from build123d import *

# Parameters (mm, degrees)
SKETCH1_W            = 275
SKETCH1_H            = 33
BOSS_EXTRUDE1_DEPTH  = 12
CUT_EXTRUDE1_REACH   = 141.005
SKETCH2_R            = 11
SKETCH2_R_2          = 2.5
BOSS_EXTRUDE2_DEPTH  = 12
CUT_EXTRUDE2_REACH   = 250.863
SKETCH4_R            = 2.5
CUT_EXTRUDE3_REACH   = 278.522
SKETCH5_W            = 14
SKETCH5_H            = 6
FILLET1_R            = 2
FILLET1_OF_MIRROR2_R = 2
CHAMFER1_SIZE        = 10
CUT_EXTRUDE4_REACH   = 278.522
SKETCH6_W            = 12
SKETCH6_H            = 30
CHAMFER2_SIZE        = 10


with BuildPart() as part:
    # Sketch1 → Boss-Extrude1 (new body)
    with BuildSketch(Plane.XY):
        Rectangle(SKETCH1_W, SKETCH1_H)
    extrude(amount=BOSS_EXTRUDE1_DEPTH)

    # Sketch2 → Cut-Extrude1 (cut, up to next)
    with BuildSketch(Plane.XY.offset(12), mode=Mode.PRIVATE) as cut_extrude1_sk1:
        with Locations((0, 1)):
            Circle(SKETCH2_R)
    cut_extrude1_tool1 = extrude(cut_extrude1_sk1.sketch, amount=-CUT_EXTRUDE1_REACH, mode=Mode.PRIVATE) & part.part
    # Sketch2 → Cut-Extrude1 (cut, up to next)
    with BuildSketch(Plane.XY.offset(12), mode=Mode.PRIVATE) as cut_extrude1_sk2:
        with Locations((-16.5, 1)):
            Circle(SKETCH2_R_2)
    cut_extrude1_tool2 = extrude(cut_extrude1_sk2.sketch, amount=-CUT_EXTRUDE1_REACH, mode=Mode.PRIVATE) & part.part
    # Sketch2 → Cut-Extrude1 (cut, up to next)
    with BuildSketch(Plane.XY.offset(12), mode=Mode.PRIVATE) as cut_extrude1_sk3:
        with Locations((16.5, 1)):
            Circle(SKETCH2_R_2)
    cut_extrude1_tool3 = extrude(cut_extrude1_sk3.sketch, amount=-CUT_EXTRUDE1_REACH, mode=Mode.PRIVATE) & part.part
    add(cut_extrude1_tool1.solids().sort_by_distance((0, 1, 12))[0], mode=Mode.SUBTRACT)
    add(cut_extrude1_tool2.solids().sort_by_distance((-16.5, 1, 12))[0], mode=Mode.SUBTRACT)
    add(cut_extrude1_tool3.solids().sort_by_distance((16.5, 1, 12))[0], mode=Mode.SUBTRACT)

    # Sketch3 → Boss-Extrude2 (add)
    with BuildSketch(Plane.XY.offset(12)):
        Polygon((-210, 16.5), (210, 16.5), (210, 179.5), (183, 179.5), (183, 46.5), (-183, 46.5), (-183, 179.5), (-210, 179.5), align=None)
    extrude(amount=-BOSS_EXTRUDE2_DEPTH)

    # Sketch4 → Cut-Extrude2 (cut, up to next)
    with BuildSketch(Plane(origin=(0, 46.5, 0), x_dir=(1, 0, 0), z_dir=(0, 1, 0)), mode=Mode.PRIVATE) as cut_extrude2_sk1:
        with Locations(Location((-144, -6, 0), (0, 0, 270))):
            Circle(SKETCH4_R)
    cut_extrude2_tool1 = extrude(cut_extrude2_sk1.sketch, amount=-CUT_EXTRUDE2_REACH, mode=Mode.PRIVATE) & part.part
    # Sketch4 → Cut-Extrude2 (cut, up to next)
    with BuildSketch(Plane(origin=(0, 46.5, 0), x_dir=(1, 0, 0), z_dir=(0, 1, 0)), mode=Mode.PRIVATE) as cut_extrude2_sk2:
        with Locations(Location((-176, -6, 0), (0, 0, 270))):
            Circle(SKETCH4_R)
    cut_extrude2_tool2 = extrude(cut_extrude2_sk2.sketch, amount=-CUT_EXTRUDE2_REACH, mode=Mode.PRIVATE) & part.part
    cut_extrude2_1 = cut_extrude2_tool1.solids().sort_by_distance((-144, 46.5, 6))[0]
    add(cut_extrude2_1, mode=Mode.SUBTRACT)
    cut_extrude2_2 = cut_extrude2_tool2.solids().sort_by_distance((-176, 46.5, 6))[0]
    add(cut_extrude2_2, mode=Mode.SUBTRACT)
    cut_extrude2 = cut_extrude2_1 + cut_extrude2_2  # Cut-Extrude2 as one shape, for the pattern or mirror that repeats it

    # Mirror1: Cut-Extrude2 across plane
    add(cut_extrude2.mirror(Plane(origin=(0, 0, 0), x_dir=(0, 0, 1), z_dir=(1, 0, 0))), mode=Mode.SUBTRACT)

    # Sketch5 → Cut-Extrude3 (cut, up to next)
    with BuildSketch(Plane.XY.offset(12), mode=Mode.PRIVATE) as cut_extrude3_sk1:
        with Locations((-176, 43.5)):
            Rectangle(SKETCH5_W, SKETCH5_H)
    cut_extrude3_tool1 = extrude(cut_extrude3_sk1.sketch, amount=-CUT_EXTRUDE3_REACH, mode=Mode.PRIVATE) & part.part
    # Sketch5 → Cut-Extrude3 (cut, up to next)
    with BuildSketch(Plane.XY.offset(12), mode=Mode.PRIVATE) as cut_extrude3_sk2:
        with Locations((-144, 43.5)):
            Rectangle(SKETCH5_W, SKETCH5_H)
    cut_extrude3_tool2 = extrude(cut_extrude3_sk2.sketch, amount=-CUT_EXTRUDE3_REACH, mode=Mode.PRIVATE) & part.part
    cut_extrude3_1 = cut_extrude3_tool1.solids().sort_by_distance((-176, 43.5, 12))[0]
    add(cut_extrude3_1, mode=Mode.SUBTRACT)
    cut_extrude3_2 = cut_extrude3_tool2.solids().sort_by_distance((-144, 43.5, 12))[0]
    add(cut_extrude3_2, mode=Mode.SUBTRACT)
    cut_extrude3 = cut_extrude3_1 + cut_extrude3_2  # Cut-Extrude3 as one shape, for the pattern or mirror that repeats it

    # Fillet1
    fillet1_edges = [part.edges().sort_by_distance(p)[0] for p in [
        (-169, 40.5, 6),
        (-183, 40.5, 6),
        (-137, 40.5, 6),
        (-151, 40.5, 6),
    ]]
    fillet(fillet1_edges, radius=FILLET1_R)

    # Mirror2: Cut-Extrude3 across plane
    add(cut_extrude3.mirror(Plane(origin=(0, 0, 0), x_dir=(0, 0, 1), z_dir=(1, 0, 0))), mode=Mode.SUBTRACT)

    # Fillet1 of Mirror2
    fillet1_of_mirror2_edges = [part.edges().sort_by_distance(p)[0] for p in [
        (169, 40.5, 6),
        (183, 40.5, 6),
        (137, 40.5, 6),
        (151, 40.5, 6),
    ]]
    fillet(fillet1_of_mirror2_edges, radius=FILLET1_OF_MIRROR2_R)

    # Chamfer1
    chamfer1_edges = [part.edges().sort_by_distance(p)[0] for p in [
        (210, 16.5, 6),
        (-210, 16.5, 6),
    ]]
    chamfer(chamfer1_edges, length=CHAMFER1_SIZE)

    # Sketch6 → Cut-Extrude4 (cut, up to next)
    with BuildSketch(Plane.XY.offset(12), mode=Mode.PRIVATE) as cut_extrude4_sk1:
        with Locations((-194, 164.5)):
            Rectangle(SKETCH6_W, SKETCH6_H)
    cut_extrude4_tool1 = extrude(cut_extrude4_sk1.sketch, amount=-CUT_EXTRUDE4_REACH, mode=Mode.PRIVATE) & part.part
    cut_extrude4 = cut_extrude4_tool1.solids().sort_by_distance((-194, 164.5, 12))[0]
    add(cut_extrude4, mode=Mode.SUBTRACT)

    # Mirror3: Cut-Extrude4 across plane
    add(cut_extrude4.mirror(Plane(origin=(0, 0, 0), x_dir=(0, 0, 1), z_dir=(1, 0, 0))), mode=Mode.SUBTRACT)

    # Chamfer2
    chamfer2_edges = [part.edges().sort_by_distance(p)[0] for p in [
        (210, 179.5, 6),
        (-210, 179.5, 6),
    ]]
    chamfer(chamfer2_edges, length=CHAMFER2_SIZE - 0.0001)  # a hair under: the kernel refuses the full size


solid = part.part
Build history of the part. All positions in model axes, mm. A direction names the side the tool comes from. Round coordinates to 2 decimals unless told otherwise and drop trailing zeros. Write each loop counter-clockwise with the first axis right and the second up, starting at its lowest first coordinate (ties: lowest second). Pieces come first, ordered by that corner, then holes. Notation, with made-up numbers: (36.5, 24) -> (54.5, 24) arc R32 cw to (54.5, 55) -> close; hole circle Ø5 at (51, 78.5). An arc over 180 degrees is marked (long way). Use one line per item in the form item = value.
Q1. Band-saw the part on C-C, the plane z = 6. State how many separate pieces and enclosed holes the cut face has, then the cut area to 3 significant figures.
Conclusion:
separate_pieces = 5
enclosed_holes = 3
area = 26,700 mm²
Q2. Drop flat-ended pins along their axis: P1, Ø6.5, axis at x = -144, z = 6, coming from the +Y side; P2, Ø1.5, axis at x = 134.5, z = 2.5, coming from the +Y side. Give the stop position or say it passes through.
Conclusion:
P1 = 40.5
P2 = 46.5
Q3. Tool access for faces 4 (the flat face through (168, 16.5, 6)), 5 (the flat face through (-137.5, 0, 6)), 6 (the flat face through (146.3, 40.5, 7.4)), 7 (the flat face through (-204.9, 174.6, 6.1)): list every direction of +Z, -Z, +X, -X, +Y, -Y with a clear straight run to the whole face (end or side of a thin tool).
Conclusion:
face_4 = +Z, -Z, +X, -Y
face_5 = +Z, -Z, -X, -Y
face_6 = +Z, -Z, +Y
face_7 = +Z, -Z, -X, +Y
Q4. Band-saw the part on A-A, the plane y = 89. Write the cut outline in (x, z).
Conclusion:
outline = (-210, 0) -> (-183, 0) -> (-183, 12) -> (-210, 12) -> close; (183, 0) -> (210, 0) -> (210, 12) -> (183, 12) -> close
Q5. Band-saw the part on B-B, the plane x = 0. Write the cut outline in (y, z).
Conclusion:
outline = (-16.5, 0) -> (-10, 0) -> (-10, 12) -> (-16.5, 12) -> close; (12, 0) -> (46.5, 0) -> (46.5, 12) -> (12, 12) -> close
Q6. Drill centre lines: L1, parallel to X at y = 30, z = 6; L2, parallel to Z at x = 176, y = 26; L3, parallel to X at y = 0.5, z = 0.5. Where is each one in solid material? Low to high.
Conclusion:
L1 = -210 to -178.5, -173.5 to -146.5, -141.5 to 141.5, 146.5 to 173.5, 178.5 to 210
L2 = 0 to 3.5, 8.5 to 12
L3 = -137.5 to -18.95, -14.05 to -10.99, 10.99 to 14.05, 18.95 to 137.5
Q7. Band-saw the part on D-D, the plane x = 86.5. Write the cut outline in (y, z).
Conclusion:
outline = (-16.5, 0) -> (46.5, 0) -> (46.5, 12) -> (-16.5, 12) -> close
Q8. Two-plate mould, pull along Y, no slides. Class faces 1 (the cylindrical face through (-2.38, -9.74, 6.08)), 2 (the flat face through (-2, -16.5, 6)), 3 (the flat face through (194, 149.5, 6)): released by +Y, released by -Y, zero draft, split by the parting line, or undercut.
Conclusion:
face_1 = undercut
face_2 = released by -Y
face_3 = released by +Y
